Model file for the job. Use its own axes, mm. Face numbers are marked on the shaded views. A direction names the side the tool comes from. Give positions to 0.01 mm unless a question says otherwise; leave off trailing zeros. Write each loop counter-clockwise with the first axis right and the second up, starting at its lowest first coordinate (ties: lowest second). Pieces come first, ordered by that corner, then holes. Notation, with made-up numbers: (16.25, 42.25) - (43.25, 42.25) arc R33 cw to (43.25, 76.25) - close; hole circle Ø5 at (-15.75, -15). An arc over 180 degrees is marked (long way). Use a Markdown table: item, result. Add a question column.
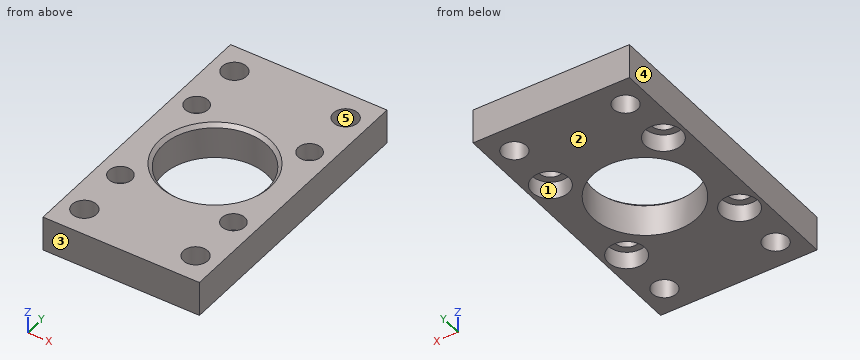
Autodesk Inventor part; units mm, degrees
ref_plane "FDT_MOUNT_XY" through (0, 0, 10) normal (0, 0, 1) x (0, 1, 0)
ref_plane "FDT_MOUNT_YZ" through (0, 0, 10) normal (0, 1, 0) x (-1, 0, 0)
ref_plane "FDT_MOUNT_ZX" through (0, 0, 10) normal (-1, 0, 0) x (0, 0, 1)
sketch "Skizze_1" plane through (0, 0, 0) normal (0, 0, 1) x (1, 0, 0)
  line L0 (-22.5, 40) -> (-22.5, -40)
  line L1 (-22.5, -40) -> (22.5, -40)
  line L2 (22.5, -40) -> (22.5, 40)
  line L3 (22.5, 40) -> (-22.5, 40)
  circle A0 centre (16, 32) radius 3.5
  circle A1 centre (16, -32) radius 3.5
  circle A2 centre (-16, 32) radius 3.5
  circle A3 centre (-16, -32) radius 3.5
extrude "Extrusion1" add sketch "Skizze_1" along normal blind 10
sketch "Skizze_2_ALT_Drilling_1" plane through (0, 0, 0) normal (1, 0, 0) x (0, 1, 0)
  line L0 (0, 0) -> (0, 10)
  line L1 (0, 10) -> (16, 10)
  line L2 (16, 10) -> (15, 9)
  line L3 (15, 9) -> (15, 0)
  line L4 (15, 0) -> (0, 0)
  line L5 (0, 0) -> (0, 10)
revolve "Revolution1" cut sketch "Skizze_2_ALT_Drilling_1" angle 360 about axis through (0, 0, 0) along (0, 0, -1)
sketch "Skizze_3_ALT_Drilling_2" plane through (16.25, 0, 0) normal (1, 0, 0) x (0, 0, -1)
  line L0 (0, 16.25) -> (-10, 16.25)
  line L1 (-10, 16.25) -> (-10, 19.55)
  line L2 (-10, 19.55) -> (-5, 19.55)
  line L3 (-5, 19.55) -> (-5, 21.5)
  line L4 (-5, 21.5) -> (0, 21.5)
  line L5 (0, 21.5) -> (0, 16.25)
  line L6 (0, 16.25) -> (-10, 16.25)
revolve "Revolution2" cut sketch "Skizze_3_ALT_Drilling_2" angle 360 about axis through (16.25, 16.25, 0) along (0, 0, -1)
sketch "Muster_1_SKETCH_1" plane through (-16.25, 0, 0) normal (1, 0, 0) x (0, 0, -1)
  line L0 (0, 16.25) -> (-10, 16.25)
  line L1 (-10, 16.25) -> (-10, 19.55)
  line L2 (-10, 19.55) -> (-5, 19.55)
  line L3 (-5, 19.55) -> (-5, 21.5)
  line L4 (-5, 21.5) -> (0, 21.5)
  line L5 (0, 21.5) -> (0, 16.25)
  line L6 (0, 16.25) -> (-10, 16.25)
sketch "Muster_1_SKETCH_2" plane through (16.25, 0, 0) normal (1, 0, 0) x (0, 0, -1)
  line L0 (0, -16.25) -> (-10, -16.25)
  line L1 (-10, -16.25) -> (-10, -12.95)
  line L2 (-10, -12.95) -> (-5, -12.95)
  line L3 (-5, -12.95) -> (-5, -11)
  line L4 (-5, -11) -> (0, -11)
  line L5 (0, -11) -> (0, -16.25)
  line L6 (0, -16.25) -> (-10, -16.25)
sketch "Muster_1_SKETCH_3" plane through (-16.25, 0, 0) normal (1, 0, 0) x (0, 0, -1)
  line L0 (0, -16.25) -> (-10, -16.25)
  line L1 (-10, -16.25) -> (-10, -12.95)
  line L2 (-10, -12.95) -> (-5, -12.95)
  line L3 (-5, -12.95) -> (-5, -11)
  line L4 (-5, -11) -> (0, -11)
  line L5 (0, -11) -> (0, -16.25)
  line L6 (0, -16.25) -> (-10, -16.25)
revolve "Revolution3" cut sketch "Muster_1_SKETCH_1" angle 360 about axis through (-16.25, 16.25, 0) along (0, 0, -1)
revolve "Revolution4" cut sketch "Muster_1_SKETCH_2" angle 360 about axis through (16.25, -16.25, 0) along (0, 0, -1)
revolve "Revolution5" cut sketch "Muster_1_SKETCH_3" angle 360 about axis through (-16.25, -16.25, 0) along (0, 0, -1)
ref_plane "FDT_MOUNT_XY" through (0, 0, 10) normal (0, 0, 1) x (0, 1, 0)
ref_plane "FDT_MOUNT_YZ" through (0, 0, 10) normal (0, 1, 0) x (-1, 0, 0)
ref_plane "FDT_MOUNT_ZX" through (0, 0, 10) normal (-1, 0, 0) x (0, 0, 1)
ref_plane "FNC_1_XY" through (0, 0, 5) normal (0, 0, 1) x (1, 0, 0)
ref_plane "FNC_1_YZ" through (0, 0, 5) normal (1, 0, 0) x (0, 1, 0)
ref_plane "FNC_1_ZX" through (0, 0, 5) normal (0, 1, 0) x (0, 0, 1)
ref_plane "FNC_2_3_XY" through (0, 0, 10) normal (0, 0, 1) x (1, 0, 0)
ref_plane "FNC_2_3_YZ" through (0, 0, 10) normal (1, 0, 0) x (0, 1, 0)
ref_plane "FNC_2_3_ZX" through (0, 0, 10) normal (0, 1, 0) x (0, 0, 1)
ref_plane "FNC_Schraube_1_XY" through (-16.25, 16.25, 5) normal (0, 0, 1) x (1, 0, 0)
ref_plane "FNC_Schraube_1_YZ" through (-16.25, 16.25, 5) normal (1, 0, 0) x (0, 1, 0)
ref_plane "FNC_Schraube_1_ZX" through (-16.25, 16.25, 5) normal (0, 1, 0) x (0, 0, 1)
ref_plane "FNC_Schraube_2_XY" through (16.25, 16.25, 5) normal (0, 0, 1) x (1, 0, 0)
ref_plane "FNC_Schraube_2_YZ" through (16.25, 16.25, 5) normal (1, 0, 0) x (0, 1, 0)
ref_plane "FNC_Schraube_2_ZX" through (16.25, 16.25, 5) normal (0, 1, 0) x (0, 0, 1)
ref_plane "FNC_Schraube_3_XY" through (-16.25, -16.25, 5) normal (0, 0, 1) x (1, 0, 0)
ref_plane "FNC_Schraube_3_YZ" through (-16.25, -16.25, 5) normal (1, 0, 0) x (0, 1, 0)
ref_plane "FNC_Schraube_3_ZX" through (-16.25, -16.25, 5) normal (0, 1, 0) x (0, 0, 1)
ref_plane "FNC_Schraube_4_XY" through (16.25, -16.25, 5) normal (0, 0, 1) x (1, 0, 0)
ref_plane "FNC_Schraube_4_YZ" through (16.25, -16.25, 5) normal (1, 0, 0) x (0, 1, 0)
ref_plane "FNC_Schraube_4_ZX" through (16.25, -16.25, 5) normal (0, 1, 0) x (0, 0, 1)
ref_plane "P17_XY" through (16, 32, 10) normal (0, 0, 1) x (1, 0, 0)
ref_plane "P17_YZ" through (16, 32, 10) normal (1, 0, 0) x (0, 1, 0)
ref_plane "P17_ZX" through (16, 32, 10) normal (0, 1, 0) x (0, 0, 1)
ref_plane "P18_XY" through (16, -32, 10) normal (0, 0, 1) x (1, 0, 0)
ref_plane "P18_YZ" through (16, -32, 10) normal (1, 0, 0) x (0, 1, 0)
ref_plane "P18_ZX" through (16, -32, 10) normal (0, 1, 0) x (0, 0, 1)
ref_plane "P19_XY" through (-16, -32, 10) normal (0, 0, 1) x (1, 0, 0)
ref_plane "P19_YZ" through (-16, -32, 10) normal (1, 0, 0) x (0, 1, 0)
ref_plane "P19_ZX" through (-16, -32, 10) normal (0, 1, 0) x (0, 0, 1)
ref_plane "P20_XY" through (-16, 32, 10) normal (0, 0, 1) x (1, 0, 0)
ref_plane "P20_YZ" through (-16, 32, 10) normal (1, 0, 0) x (0, 1, 0)
ref_plane "P20_ZX" through (-16, 32, 10) normal (0, 1, 0) x (0, 0, 1)
properties part number "174376 FNC-32---(F)"
(1) Two-plate mould, pull along Y, no slides. Class the marked faces 3, 4 and 5: +Y half, -Y half, draft (parallel to the pull), parting line (faces both ways), or undercut.
(2) Probe probe 1 along X at (y, z) = (-16.25, 6.1); probe 2 along X at (y, z) = (-16.25, 2.25); probe 3 along Y at (x, z) = (16, 3.5). List the from-to ranges inside material, lowest first. Write a range as [from, to].
(3) Band-saw the part on A-A (z = 2.25). Give the number of separate pieces and of enclosed holes in the cut face, then the cut area to 3 significant figures.
(4) Band-saw the part on B-B (y = -32). Write the cut outline in (x, z).
(5) Flat gauge pin, fed straight in: pin 1 (8.5 mm diameter, centred on x = 16.25, y = 16.25, fed in from -Z). Where does the tip first touch, or does it go through?
(6) Which spindle directions (+Z, -Z, +X, -X, +Y, -Y) get a long thin tool onto all of the face, cutting with end or side? Do the marked faces 1 and 2. Say none if no direction does.
Model answer:
| question | item | result |
|---|---|---|
| 1 | face 3 | -Y half |
| 1 | face 4 | draft |
| 1 | face 5 | undercut |
| 2 | probe 1 | x = [-22.5, -19.55], [-12.95, 12.95], [19.55, 22.5] |
| 2 | probe 2 | x = [-22.5, -21.5], [-11, 11], [21.5, 22.5] |
| 2 | probe 3 | y = [-40, -35.5], [-28.5, -21.49], [-11.01, 11.01], [21.49, 28.5], [35.5, 40] |
| 3 | separate pieces | 1 |
| 3 | enclosed holes | 9 |
| 3 | area | 2,390 mm^2 |
| 4 | outline | (-22.5, 0) - (-19.5, 0) - (-19.5, 10) - (-22.5, 10) - close; (-12.5, 0) - (12.5, 0) - (12.5, 10) - (-12.5, 10) - close; (19.5, 0) - (22.5, 0) - (22.5, 10) - (19.5, 10) - close |
| 5 | pin 1 | stops at z = 5 |
| 6 | face 1 | -Z |
| 6 | face 2 | -Z, +X, -X, +Y, -Y |
